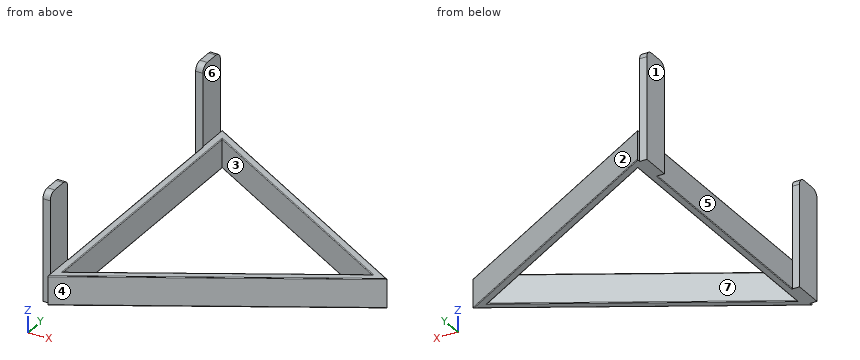
```python
from build123d import *

# Parameters (mm, degrees)
F1_DEPTH = 40
F3_DEPTH = 10
F4_R     = 1


with BuildPart() as f1:
    # F0 (on Top) → F1 (new body)
    with BuildSketch(Plane.XY):
        Polygon((-346.4101615138, -200), (0, 0), (-346.4101615138, 200), align=None)
        Polygon((-336.4101615138, 182.6794919243), (-20, 0), (-336.4101615138, -182.6794919243), align=None, mode=Mode.SUBTRACT)
    extrude(amount=F1_DEPTH)

    # F2 (on face) → F3 (join)
    with BuildSketch(Plane(origin=(-346.4101615138, 0, 0), x_dir=(0, -1, 0), z_dir=(-1, 0, 0))):
        with BuildLine():
            Line((-195, 140), (-195, 0))
            Line((-195, 0), (-155, 0))
            Line((-155, 0), (-155, 140))
            ThreePointArc((-155, 140), (-157.9289321881, 147.0710678119), (-165, 150))
            Line((-165, 150), (-185, 150))
            ThreePointArc((-185, 150), (-192.0710678119, 147.0710678119), (-195, 140))
        make_face()
        with BuildLine():
            Line((155, 0), (195, 0))
            Line((195, 0), (195, 140))
            ThreePointArc((195, 140), (192.0710678119, 147.0710678119), (185, 150))
            Line((185, 150), (165, 150))
            ThreePointArc((165, 150), (157.9289321881, 147.0710678119), (155, 140))
            Line((155, 140), (155, 0))
        make_face()
    extrude(amount=F3_DEPTH)

    # F4
    f4_edges = [f1.edges().sort_by_distance(p)[0] for p in [
        (-346.410162, 0, 40),
        (-178.205081, 91.339746, 40),
        (-173.205081, 100, 40),
        (-173.205081, -100, 40),
        (-178.205081, -91.339746, 40),
        (-336.410162, 0, 40),
        (-173.205081, -100, 0),
        (-173.205081, 100, 0),
        (-346.410162, 0, 0),
        (-178.205081, -91.339746, 0),
        (-178.205081, 91.339746, 0),
        (-336.410162, 0, 0),
    ]]
    fillet(f4_edges, radius=F4_R)


solid = f1.part
```
Geometry check sheet. Reference: the model listing, model coordinates, mm. Face numbers are marked on the shaded views. A direction names the side the tool comes from. Coordinates: 2 decimals unless noted, no trailing zeros. Order: outer loops, then holes, each group sorted by start corner. A loop starts at its lowest first (then second) coordinate and runs counter-clockwise, first axis right, second up. Notation, with made-up numbers: (19, -26) - (75, -26) arc R34 ccw to (75, 13) - close; hole circle Ø2 at (-29.5, 78.5). An arc over 180 degrees is marked (long way). Answer in a Markdown table with one row per item. Add a question column.
1. Draft check along X on the marked faces 1, 2 and 3. Enter one of: +X half, -X half, draft (parallel to the pull), parting line (faces both ways), or undercut.
2. Access from +Z, -Z, +X, -X, +Y, -Y to the whole of each face (thin tool, end or side, straight path). Record for the marked faces 4, 5, 6 and 7.
3. Section check B-B (z = 34). Enter the section's corners in (x, y), plus the area to 3 significant figures.
4. Gauge pin test, flat ends, axial feed: pin 1 Ø11.5 at (y, z) = (-17, 17.5) entering from +X; pin 2 Ø9 at (x, z) = (-353, 104.5) entering from -Y; pin 3 Ø8 at (x, z) = (-111.5, 37) entering from -Y. Record the tip position at first contact, or that the pin passes through.
5. Section check A-A (z = 102.5). Enter the section's corners in (x, y).
6. Material ranges on L1, parallel to X at y = -166.5, z = 88.5; L2, parallel to X at y = -42, z = 11.5; L3, parallel to Y at x = -308.5, z = 12, recorded low to high. Write a range as [from, to].
Data:
| question | item | result |
|---|---|---|
| 1 | face 1 | -X half |
| 1 | face 2 | +X half |
| 1 | face 3 | undercut |
| 2 | face 4 | +Z, -Z, +X, -Y |
| 2 | face 5 | +Z, -Z, -X |
| 2 | face 6 | +Z, +X, +Y, -Y |
| 2 | face 7 | +Z, -Z |
| 3 | outline | (-356.41, -195) - (-346.41, -195) - (-346.41, -200) - (0, 0) - (-346.41, 200) - (-346.41, 195) - (-356.41, 195) - (-356.41, 155) - (-346.41, 155) - (-346.41, -155) - (-356.41, -155) - close; hole (-336.41, -182.68) - (-20, 0) - (-336.41, 182.68) - close |
| 3 | area | 12,300 mm² |
| 4 | pin 1 | stops at x = -19.49 |
| 4 | pin 2 | stops at y = -195 |
| 4 | pin 3 | stops at y = -66.68 |
| 5 | outline | (-356.41, -195) - (-346.41, -195) - (-346.41, -155) - (-356.41, -155) - close; (-356.41, 155) - (-346.41, 155) - (-346.41, 195) - (-356.41, 195) - close |
| 6 | L1 | x = [-356.41, -346.41] |
| 6 | L2 | x = [-346.41, -336.41], [-92.75, -72.75] |
| 6 | L3 | y = [-178.11, -166.57], [166.57, 178.11] |
